Drawing for the job (mm, zero at the part's lowest x, y, z). Give positions to 0.01 mm unless a question says otherwise; leave off trailing zeros. Order: outer loops, then holes, each group sorted by start corner. A loop starts at its lowest first (then second) coordinate and runs counter-clockwise, first axis right, second up. Notation, with made-up numbers: (-24, 88.5) - (34, 88.5) arc R28 ccw to (34, 114.5) - close; hole circle Ø1 at (48, -38.5). An arc over 180 degrees is marked (long way). Use a Markdown table: item, result.
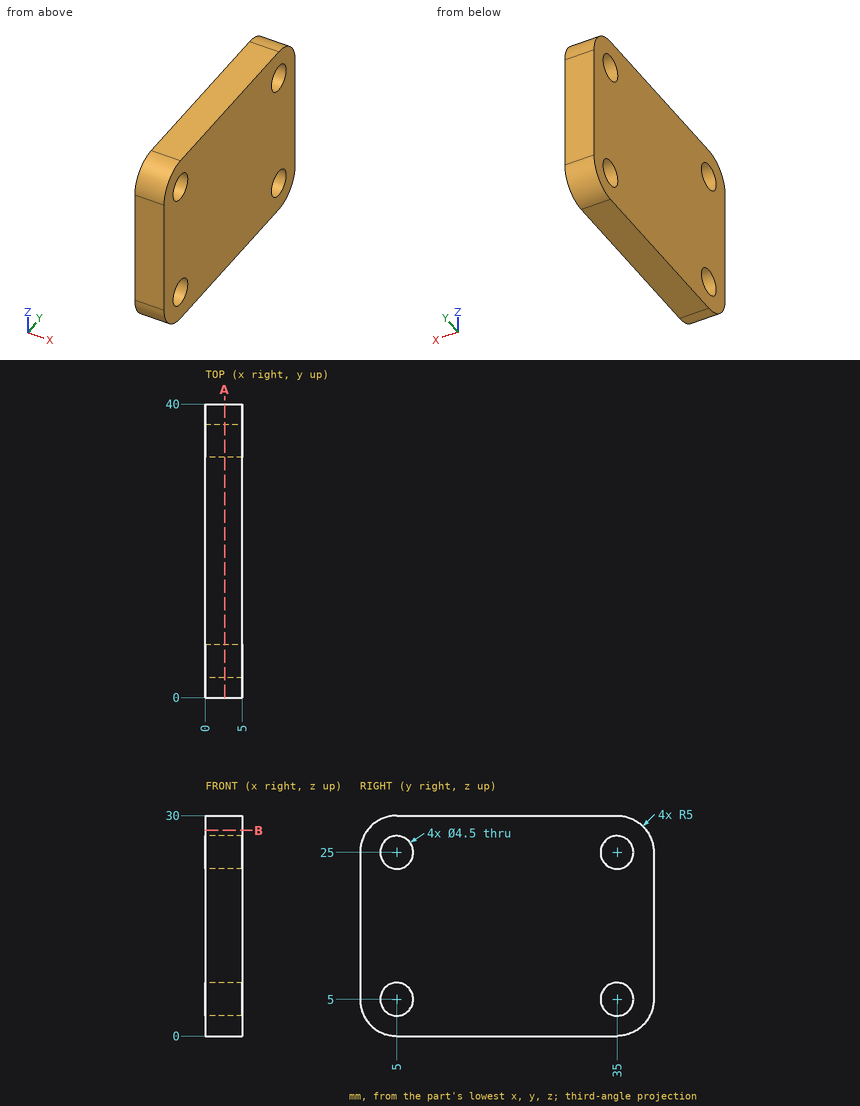
1) Wall check: line 1 (Z direction, x = 2.9, y = 5); line 2 (Y direction, x = 4.7, z = 4.25); line 3 (Y direction, x = 2.35, z = 5.25). Give the ranges that are in metal, low to high. Write a range as from..to.
Computed:
| item | result |
|---|---|
| line 1 | z = 0..2.75, 7.25..22.75, 27.25..30 |
| line 2 | y = 0.06..2.88, 7.12..32.88, 37.12..39.94 |
| line 3 | y = 0..2.76, 7.24..32.76, 37.24..40 |
2) Slice it at A-A (x = 2.65). Write the cut outline in (y, z), and give its area (3 significant figures).
Computed:
| item | result |
|---|---|
| outline | (0, 5) arc R5 ccw to (5, 0) - (35, 0) arc R5 ccw to (40, 5) - (40, 25) arc R5 ccw to (35, 30) - (5, 30) arc R5 ccw to (0, 25) - close; hole circle Ø4.5 at (5, 5); hole circle Ø4.5 at (5, 25); hole circle Ø4.5 at (35, 5); hole circle Ø4.5 at (35, 25) |
| area | 1,110 mm² |
3) Slice it at B-B (z = 28). Write the cut outline in (x, y).
Computed:
| item | result |
|---|---|
| outline | (0, 1) - (5, 1) - (5, 39) - (0, 39) - close |
